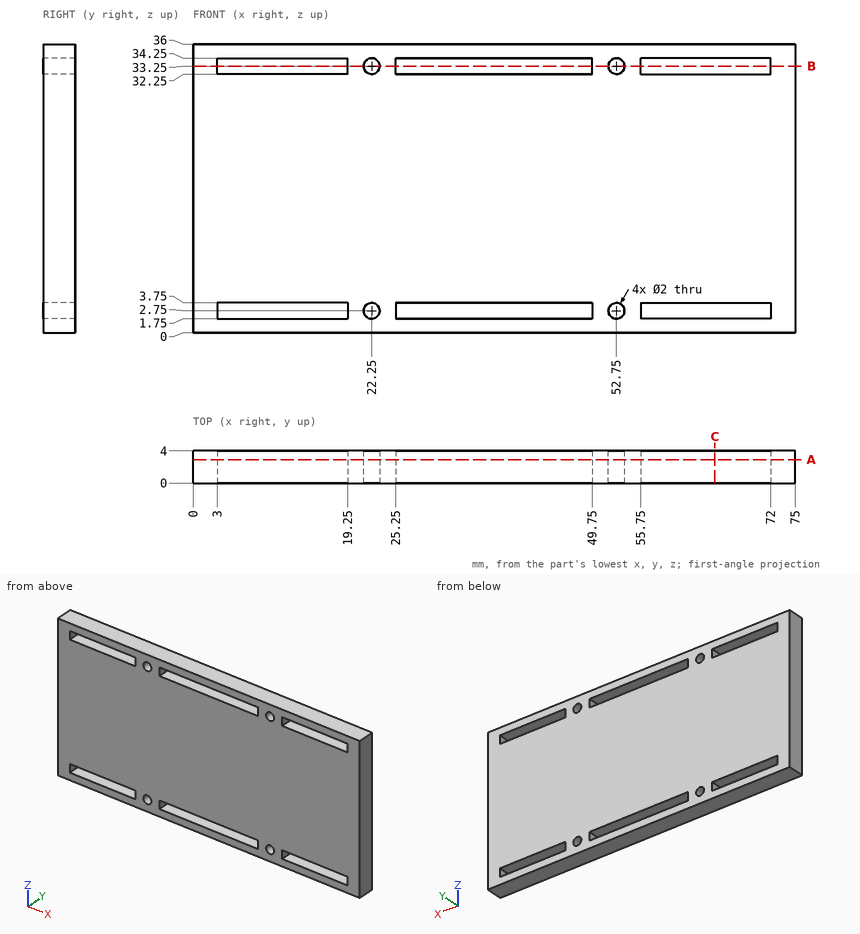
Can you work these out from the drawing? Everything is in mm from the part's minimum corner. Coordinates: 2 decimals unless noted, no trailing zeros. Loops run counter-clockwise (first coordinate to the right, second up) from the corner with the lowest first, then second, coordinate; pieces in that order, holes last.
1. For P1, Ø2.5, axis at x = 52.75, z = 33.25, coming from the +Y side; P2, Ø1.2, axis at x = 52.75, z = 2.75, coming from the +Y side, each with a flat end and sliding along its axis, tell me the tip position at first contact or that it passes through.
2. Imagine slicing it at C-C, the plane x = 65. Please give me the cut outline in (y, z), and give its area (3 significant figures).
3. Imagine slicing it at B-B, the plane z = 33.25. Please give me the cut outline in (x, y).
4. Imagine slicing it at A-A, the plane y = 2.9. Count the separate pieces of the cut face and the enclosed holes in it, and give its area (3 significant figures).
5. I need wall thicknesses on L1, parallel to X at y = 1.1, z = 2.75; L2, parallel to Z at x = 52.75, y = 2.4. Which ranges of each line are inside material? Lowest first, please.
Taken from the geometry:
1. P1: stops at y = 4
1. P2: passes through
2. outline: (0, 0) - (4, 0) - (4, 1.75) - (0, 1.75) - close; (0, 3.75) - (4, 3.75) - (4, 32.25) - (0, 32.25) - close; (0, 34.25) - (4, 34.25) - (4, 36) - (0, 36) - close
2. area: 128 mm2
3. outline: (0, 0) - (3, 0) - (3, 4) - (0, 4) - close; (19.25, 0) - (21.25, 0) - (21.25, 4) - (19.25, 4) - close; (23.25, 0) - (25.25, 0) - (25.25, 4) - (23.25, 4) - close; (49.75, 0) - (51.75, 0) - (51.75, 4) - (49.75, 4) - close; (53.75, 0) - (55.75, 0) - (55.75, 4) - (53.75, 4) - close; (72, 0) - (75, 0) - (75, 4) - (72, 4) - close
4. separate pieces: 1
4. enclosed holes: 10
4. area: 2,460 mm2
5. L1: x = 0 to 3, 19.25 to 21.25, 23.25 to 25.25, 49.75 to 51.75, 53.75 to 55.75, 72 to 75
5. L2: z = 0 to 1.75, 3.75 to 32.25, 34.25 to 36
